Source: CAD feature listing. Evaluate the final solid. Frame: model axes, mm. Face numbers are marked on the shaded views. Coordinates: 2 decimals unless noted, no trailing zeros. Loops run counter-clockwise (first coordinate to the right, second up) from the corner with the lowest first, then second, coordinate; pieces in that order, holes last. Notation, with made-up numbers: M -36.5,81.25 L -30.5,81.25 A19 cw -30.5,115.25 Z; hole C 0.5,-8.5 d3. An arc over 180 degrees is marked long. One line per question, with ' | ' between items. Start each with the question number.
1. Section query C-C, the plane z = 5.75. Output: boundary loops of the cut face in (x, y).
2. Section query D-D, the plane x = 30.5. Output: boundary loops of the cut face in (y, z).
3. Ray query, probe 1 along X at (y, z) = (0.75, 9.75); probe 2 along X at (y, z) = (2, 4.75); probe 3 along Y at (x, z) = (3.5, 8.5). Return the intervals inside material, ascending.
4. Mould query, pull axis Y, two halves, no side actions, for the marked faces 1, 2 and 3. Classes: pulls with the +Y half, pulls with the -Y half, needs draft (parallel to the pull), parting line crosses it, or undercut.
5. Pin query (flat end, axial travel): P1, Ø6, axis at x = -2, z = 10.5, coming from the +Y side; P2, Ø6, axis at x = 35.5, z = 13.5, coming from the -Y side; P3, Ø6, axis at x = 0, y = 0, coming from the +Z side; P4, Ø2, axis at x = 9, z = 10, coming from the -Y side. Return the tip coordinate at first contact, or that it passes through.
6. Section query B-B, the plane x = -2.5. Output: boundary loops of the cut face in (y, z), and give its area (3 significant figures).
7. Section query A-A, the plane y = 0. Output: boundary loops of the cut face in (x, z).
```python
from build123d import *

# Parameters (mm, degrees)
BOSS_EXTRU_1_DEPTH           = 15
ENL_V_MAT_EXTRU_1_DEPTH      = 91.360389552
ENL_V_MAT_EXTRU_1_DEPTH_BACK = 91.360389552
ESQUISSE3_R                  = 5


with BuildPart() as part:
    # Esquisse1 → Boss.-Extru.1 (new body)
    with BuildSketch(Plane.XY):
        with BuildLine():
            Line((80.596108007, 7.977760039), (0, 14))
            ThreePointArc((0, 14), (-14, 0), (0, -14))
            Line((0, -14), (80.596108007, -7.977760039))
            ThreePointArc((80.596108007, -7.977760039), (88, 0), (80.596108007, 7.977760039))
        make_face()
    extrude(amount=BOSS_EXTRU_1_DEPTH)

    # Esquisse3 → Enlèv. mat.-Extru.1 (cut, two sides: drawn at the far end of the back side and taken through both)
    with BuildSketch(Plane.XY.offset(15).offset(-ENL_V_MAT_EXTRU_1_DEPTH_BACK)):
        Circle(ESQUISSE3_R)
    extrude(amount=ENL_V_MAT_EXTRU_1_DEPTH + ENL_V_MAT_EXTRU_1_DEPTH_BACK, mode=Mode.SUBTRACT)


solid = part.part
```
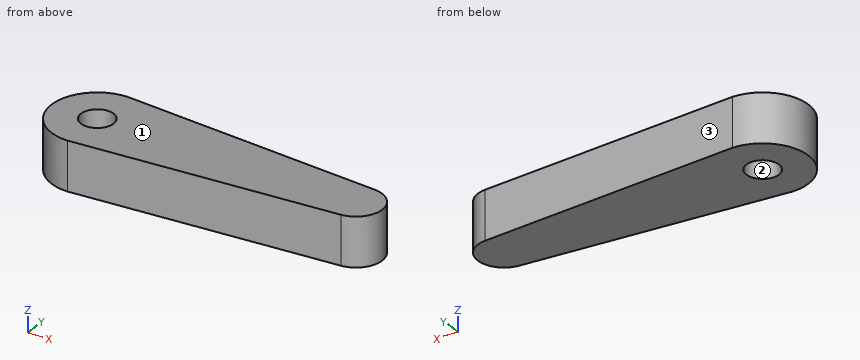
Taken from the geometry:
1) outline: M 0,-14 L 80.6,-7.98 A8 ccw 80.6,7.98 L 0,14 A14 ccw Z; hole C 0,0 d10
2) outline: M -11.72,0 L 11.72,0 L 11.72,15 L -11.72,15 Z
3) probe 1: -13.98 to -4.94, 4.94 to 87.96 | probe 2: -13.86 to -4.58, 4.58 to 87.75 | probe 3: -13.74 to -3.57, 3.57 to 13.74
4) face 1: needs draft | face 2: undercut | face 3: pulls with the +Y half
5) P1: y = 14 | P2: y = -11.57 | P3: through | P4: y = -13.4
6) outline: M -13.77,0 L -4.33,0 L -4.33,15 L -13.77,15 Z; M 4.33,0 L 13.77,0 L 13.77,15 L 4.33,15 Z | area: 283 mm^2
7) outline: M -14,0 L -5,0 L -5,15 L -14,15 Z; M 5,0 L 88,0 L 88,15 L 5,15 Z
